Autodesk Inventor part; units mm, degrees
ref_plane "YZ Plane" through (0, 0, 0) normal (1, 0, 0) x (0, 1, 0)
ref_plane "XZ Plane" through (0, 0, 0) normal (0, 1, 0) x (-1, 0, 0)
ref_plane "XY Plane" through (0, 0, 0) normal (0, 0, 1) x (1, 0, 0)
sketch "Sketch1" plane through (0, 0, 0) normal (0, 0, 1) x (1, 0, 0)
  line L0 (0, 104.6011) -> (0, -104.6011)
  line L1 (-8.6, 115.3268) -> (-8.6, 25.3268)
  arc A0 (-8.6, 25.3268) -> (-7.35, 22.0196) centre (-3.6, 25.3268) ccw
  arc A1 (-6.1, 18.7124) -> (-7.35, 22.0196) centre (-11.1, 18.7124) ccw
  line L2 (-6.1, 18.7124) -> (-6.1, -56.2876)
  arc A2 (-6.1, -56.2876) -> (0, -62.3876) centre (0, -56.2876) ccw
  arc A3 (-3.6, -56.2876) -> (0, -59.8876) centre (0, -56.2876) ccw
  line L3 (-3.6, -56.2876) -> (-3.6, 18.7124)
  arc A4 (-3.6, 18.7124) -> (-5.475, 23.6732) centre (-11.1, 18.7124) ccw
  arc A5 (-6.1, 25.3268) -> (-5.475, 23.6732) centre (-3.6, 25.3268) ccw
  line L4 (-6.1, 25.3268) -> (-6.1, 115.3268)
  line L5 (-8.6, 115.3268) -> (-6.1, 115.3268)
  line L6 (8.6, 115.3268) -> (8.6, 25.3268)
  arc A6 (7.35, 22.0196) -> (8.6, 25.3268) centre (3.6, 25.3268) ccw
  arc A7 (7.35, 22.0196) -> (6.1, 18.7124) centre (11.1, 18.7124) ccw
  line L7 (6.1, 18.7124) -> (6.1, -56.2876)
  arc A8 (0, -62.3876) -> (6.1, -56.2876) centre (0, -56.2876) ccw
  arc A9 (0, -59.8876) -> (3.6, -56.2876) centre (0, -56.2876) ccw
  line L8 (3.6, -56.2876) -> (3.6, 18.7124)
  arc A10 (5.475, 23.6732) -> (3.6, 18.7124) centre (11.1, 18.7124) ccw
  arc A11 (5.475, 23.6732) -> (6.1, 25.3268) centre (3.6, 25.3268) ccw
  line L9 (6.1, 25.3268) -> (6.1, 115.3268)
  line L10 (8.6, 115.3268) -> (6.1, 115.3268)
  point P0 (0, 0)
  point P1 (0, 0)
  dimension "d0" = 90
  dimension "d1" = 5
  dimension "d2" = 75
  dimension "d3" = 6.1
  dimension "d4" = 6.1
  dimension "d5" = 8.6
  dimension "d6" = 2.5
extrude "Extrusion1" add sketch "Sketch1" along normal mid plane 16
hole "Hole1" at (8.6, 107.3268, 0) direction (-1, 0, 0) diameter 6 depth 30 tip angle 118
hole "Hole2" at (8.6, 65.3268, 0) direction (-1, 0, 0) diameter 6 depth 30 tip angle 118
fillet "Fillet1" radius 8 4 edges at (7.35, 115.3268, -8) (7.35, 115.3268, 8) (-7.35, 115.3268, 8) (-7.35, 115.3268, -8)
equation "\"BendRadius\" = Thickness"
equation "\"BendReliefWidth\" = Thickness"
equation "\"BendReliefDepth\" = 0.5 * Thickness"
equation "\"MinimumRemnant\" = 2 * Thickness"
equation "\"TransitionRadius\" = BendRadius"
equation "\"JacobiRadiusSize\" = BendRadius"
equation "\"GapSize\" = Thickness"
properties material "Iron, Gray"
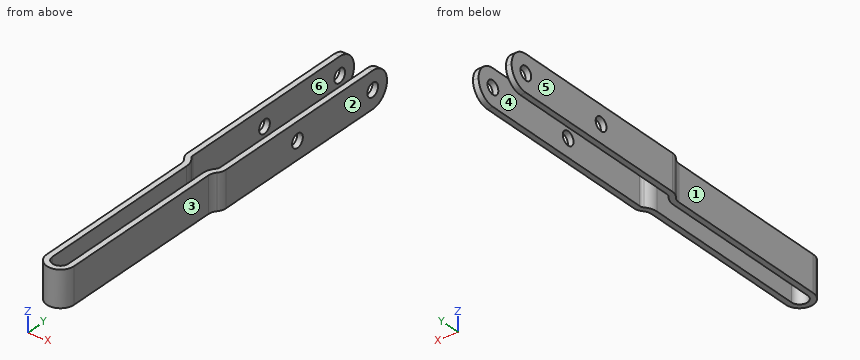
Work out the finished part from the listing and answer in its coordinate system (mm). Face numbers are marked on the shaded views. A direction names the side the tool comes from. Give positions to 0.01 mm unless a question says otherwise; leave off trailing zeros. Order: outer loops, then holes, each group sorted by start corner. A loop starts at its lowest first (then second) coordinate and runs counter-clockwise, first axis right, second up. Notation, with made-up numbers: M 64,-30.75 L 91,-30.75 A15 ccw 91,-6.75 Z; hole C 11.25,-37 d9. An arc over 180 degrees is marked long. Return JSON: item names as keys, results as strings.
Q1. Find section A-A, the plane y = 80. Write down the section's boundary in (x, z), and give its area (3 significant figures).
Answer below:
{"outline": "M -8.6,-8 L -6.1,-8 L -6.1,8 L -8.6,8 Z; M 6.1,-8 L 8.6,-8 L 8.6,8 L 6.1,8 Z", "area": "80.0 mm^2"}
Q2. Which of the six approach directions +Z, -Z, +X, -X, +Y, -Y give full straight-line access (tool end or side, diameter ignored) to the marked faces 1 and 2?
Answer below:
{"face 1": "+Z, -Z, -X, -Y", "face 2": "+Z, -Z, +X, +Y, -Y"}
Q3. Each of these flat-tipped pins is pushed along its axis until it touches: pin 1 (8 mm diameter, centred on y = -10.5, z = 0, fed in from -X); pin 2 (8 mm diameter, centred on y = -6, z = -1, fed in from +X); pin 3 (3 mm diameter, centred on y = 23, z = 0.5, fed in from +X). Where does it stop, or does it pass through?
Answer below:
{"pin 1": "stops at x = -6.1", "pin 2": "stops at x = 6.1", "pin 3": "stops at x = 8.53"}
Q4. Find the intervals of material crossed by line 1 along Y through (x, z) = (7.35, 0); line 2 along X through (y, z) = (72, 0.25); line 3 along X through (y, z) = (-11, -6.5), in increasing order. Write a range as [from, to].
Answer below:
{"line 1": "y = [22.02, 62.33], [68.33, 104.33], [110.33, 115.33]", "line 2": "x = [-8.6, -6.1], [6.1, 8.6]", "line 3": "x = [-6.1, -3.6], [3.6, 6.1]"}
Q5. The mould has two halves that part along X. Classify the marked faces 3, 4, 5 and 6: pulls with the +X half, pulls with the -X half, needs draft (parallel to the pull), parting line crosses it, or undercut.
Answer below:
{"face 3": "pulls with the +X half", "face 4": "undercut", "face 5": "pulls with the -X half", "face 6": "undercut"}
Q6. Find section C-C, the plane x = 0. Write down the section's boundary in (y, z), and give its area (3 significant figures).
Answer below:
{"outline": "M -62.39,-8 L -59.89,-8 L -59.89,8 L -62.39,8 Z", "area": "40.0 mm^2"}
Q7. Find section B-B, the plane z = -5.5. Write down the section's boundary in (x, y) (3 decimals), and give its area (3 significant figures).
Answer below:
{"outline": "M -8.6,25.327 A5 ccw -7.35,22.02 A5 cw -6.1,18.712 L -6.1,-56.288 A6.1 ccw 6.1,-56.288 L 6.1,18.712 A5 cw 7.35,22.02 A5 ccw 8.6,25.327 L 8.6,113.136 L 6.1,113.136 L 6.1,25.327 A2.5 cw 5.475,23.673 A7.5 ccw 3.6,18.712 L 3.6,-56.288 A3.6 cw -3.6,-56.288 L -3.6,18.712 A7.5 ccw -5.475,23.673 A2.5 cw -6.1,25.327 L -6.1,113.136 L -8.6,113.136 Z", "area": "888 mm^2"}
Q8. Find section D-D, the plane z = 5.75. Write down the section's boundary in (x, y) (3 decimals).
Answer below:
{"outline": "M -8.6,25.327 A5 ccw -7.35,22.02 A5 cw -6.1,18.712 L -6.1,-56.288 A6.1 ccw 6.1,-56.288 L 6.1,18.712 A5 cw 7.35,22.02 A5 ccw 8.6,25.327 L 8.6,112.889 L 6.1,112.889 L 6.1,25.327 A2.5 cw 5.475,23.673 A7.5 ccw 3.6,18.712 L 3.6,-56.288 A3.6 cw -3.6,-56.288 L -3.6,18.712 A7.5 ccw -5.475,23.673 A2.5 cw -6.1,25.327 L -6.1,112.889 L -8.6,112.889 Z"}
